Here's the drawing with two shaded views (mm, measured from the low corner). I have some questions. A direction names the side the tool comes from. Coordinates: 2 decimals unless noted, no trailing zeros. Write each loop counter-clockwise with the first axis right and the second up, starting at its lowest first coordinate (ties: lowest second). Pieces come first, ordered by that corner, then holes.
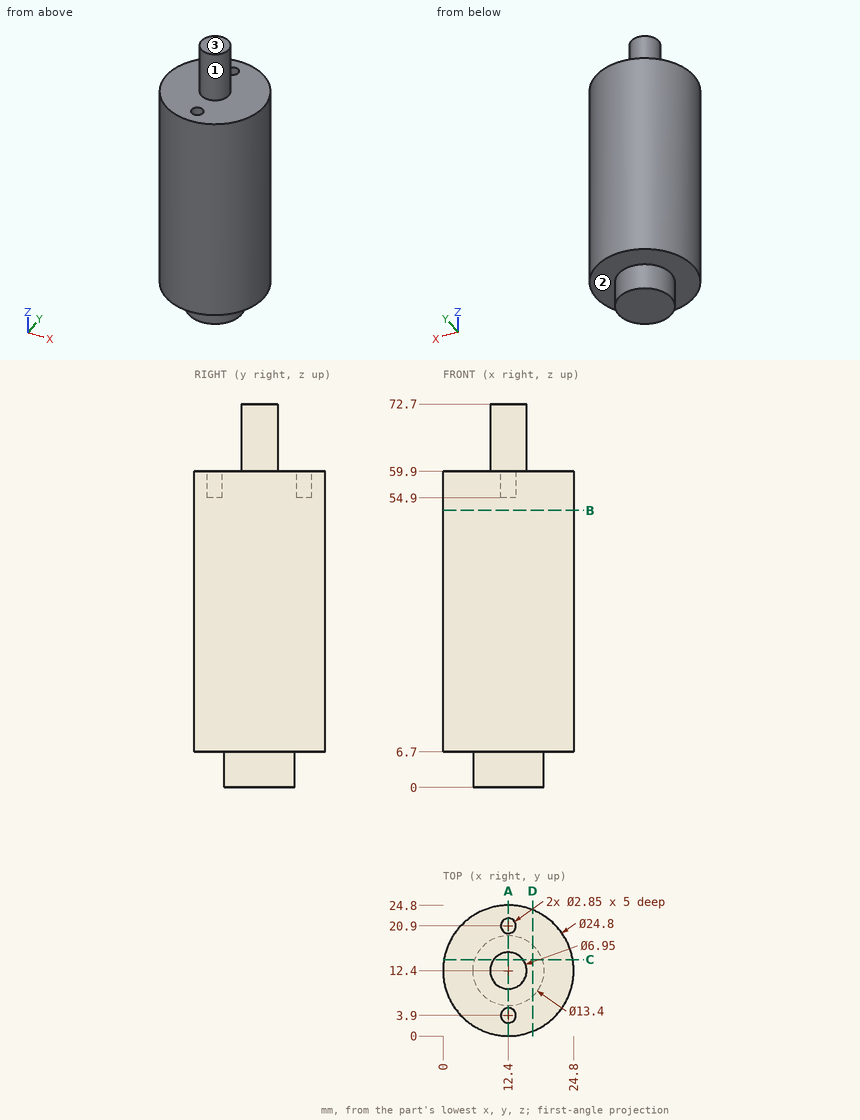
1. I want a section at D-D on x = 17. Please give me the cut outline in (y, z), plus the area to 3 significant figures.
Verdict:
outline: (0.88, 6.7) - (7.53, 6.7) - (7.53, 0) - (17.27, 0) - (17.27, 6.7) - (23.92, 6.7) - (23.92, 59.9) - (0.88, 59.9) - close
area: 1,290 mm2
2. On a 3-axis mill with a long thin cutter (end or side, diameter ignored), from which of +Z, -Z, +X, -X, +Y, -Y can I reach the whole of each face in a straight line? I mean the marked faces 1, 2 and 3. Say none if no direction works.
Verdict:
face 1: +Z
face 2: -Z
face 3: +Z, +X, -X, +Y, -Y
3. Please list where these lines run through material, in increasing order: line 1 along Y through (x, z) = (12.4, 58.2) (3 decimals); line 2 along Z through (x, y) = (21.5, 7.75); line 3 along Z through (x, y) = (10.5, 16.75).
Verdict:
line 1: y = 0 to 2.475, 5.325 to 19.475, 22.325 to 24.8
line 2: z = 6.7 to 59.9
line 3: z = 0 to 59.9
4. I want a section at B-B on z = 52.5. Please give me the cut outline in (x, y).
Verdict:
outline: circle Ø24.8 at (12.4, 12.4)
5. I want a section at A-A on x = 12.4. Please give me the cut outline in (y, z) (3 decimals).
Verdict:
outline: (0, 6.7) - (5.7, 6.7) - (5.7, 0) - (19.1, 0) - (19.1, 6.7) - (24.8, 6.7) - (24.8, 59.9) - (22.325, 59.9) - (22.325, 54.9) - (19.475, 54.9) - (19.475, 59.9) - (15.875, 59.9) - (15.875, 72.7) - (8.925, 72.7) - (8.925, 59.9) - (5.325, 59.9) - (5.325, 54.9) - (2.475, 54.9) - (2.475, 59.9) - (0, 59.9) - close
6. I want a section at C-C on y = 14.5. Please give me the cut outline in (x, z), plus the area to 3 significant figures.
Verdict:
outline: (0.18, 6.7) - (6.04, 6.7) - (6.04, 0) - (18.76, 0) - (18.76, 6.7) - (24.62, 6.7) - (24.62, 59.9) - (15.17, 59.9) - (15.17, 72.7) - (9.63, 72.7) - (9.63, 59.9) - (0.18, 59.9) - close
area: 1,460 mm2
7. For pin 1 (4 mm diameter, centred on x = 15.5, y = 18, fed in from +Z); pin 2 (7.5 mm diameter, centred on x = 14.5, y = 17, fed in from +Z); pin 3 (6 mm diameter, centred on x = 16, z = 63, fed in from -Y); pin 4 (5 mm diameter, centred on y = 7.5, z = 55, fed in from +X), each with a flat end and sliding along its axis, tell me the tip position at first contact or that it passes through.
Verdict:
pin 1: stops at z = 59.9
pin 2: stops at z = 72.7
pin 3: stops at y = 8.98
pin 4: stops at x = 24.57
